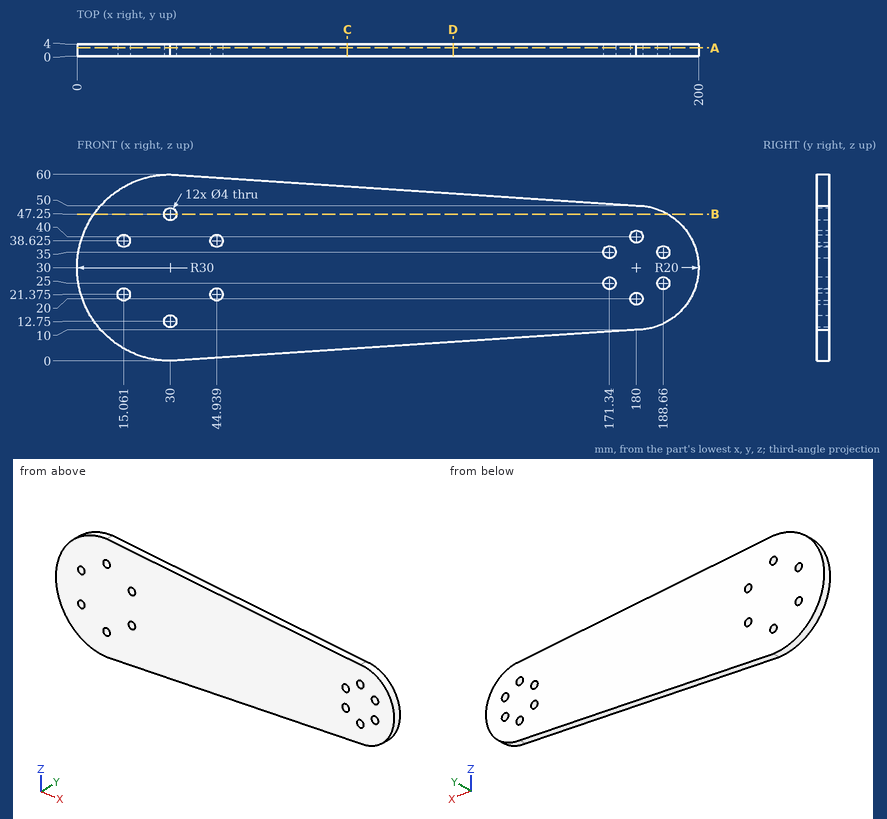
Here's the drawing with two shaded views (mm, measured from the low corner). I have some questions. Give positions to 0.01 mm unless a question says otherwise; leave off trailing zeros. Order: outer loops, then holes, each group sorted by start corner. A loop starts at its lowest first (then second) coordinate and runs counter-clockwise, first axis right, second up. Notation, with made-up numbers: (16, -21) -> (28, -21) arc R14 ccw to (28, -15) -> close; hole circle Ø5 at (21.25, 68.25). An arc over 180 degrees is marked (long way). One line per item, written item: value. Start each with the question number.
1. Imagine slicing it at C-C, the plane x = 87. List the corners of the cut face in (y, z) for me.
2. Imagine slicing it at D-D, the plane x = 121. List the corners of the cut face in (y, z) for me.
3. Imagine slicing it at A-A, the plane y = 2.75. Count the separate pieces of the cut face and the enclosed holes in it, plus the area to 3 significant figures.
4. Will these pins go through, and if not, where does the flat tip stop? pin 1 Ø6.5 at (x, z) = (171.34, 35) entering from +Y; pin 2 Ø3 at (x, z) = (180, 40) entering from +Y; pin 3 Ø1 at (y, z) = (0.5, 50) entering from -X; pin 4 Ø1.5 at (x, y) = (124, 2.5) entering from -Z.
5. Imagine slicing it at B-B, the plane z = 47.25. List the corners of the cut face in (x, y) for me (1 decimal).
6. I need wall thicknesses on probe 1 along Z at (x, y) = (190, 2.4) (1 decimal); probe 2 along X at (y, z) = (2.1, 24.5); probe 3 along X at (y, z) = (1.8, 39.5). Which ranges of each line are inside material? Lowest first, please. Write a range as from..to.
Values follow:
1. outline: (0, 3.8) -> (4, 3.8) -> (4, 56.2) -> (0, 56.2) -> close
2. outline: (0, 6.07) -> (4, 6.07) -> (4, 53.93) -> (0, 53.93) -> close
3. separate pieces: 1
3. enclosed holes: 12
3. area: 9,390 mm2
4. pin 1: stops at y = 4
4. pin 2: passes through
4. pin 3: stops at x = 7.2
4. pin 4: stops at z = 6.22
5. outline: (5.5, 0) -> (28, 0) -> (28, 4) -> (5.5, 4) -> close; (32, 0) -> (190.1, 0) -> (190.1, 4) -> (32, 4) -> close
6. probe 1: z = 12.7..23.5, 26.5..33.5, 36.5..47.3
6. probe 2: x = 0.51..169.4, 173.28..186.72, 190.6..199.23
6. probe 3: x = 1.54..13.26, 16.86..43.14, 46.74..178.06, 181.94..197.6
